Design review of the part built by this model. Coordinates are the model's own, in mm. A direction names the side the tool comes from. Coordinates: 2 decimals unless noted, no trailing zeros. Write each loop counter-clockwise with the first axis right and the second up, starting at its lowest first coordinate (ties: lowest second). Pieces come first, ordered by that corner, then holes. Notation, with made-up numbers: (44, 62.25) - (84, 62.25) arc R27 cw to (84, 81.25) - close; hole circle Ø6 at (17, 81). An arc over 180 degrees is marked (long way). Answer as a JSON object with one key per item and string values.
```python
from build123d import *

# Parameters (mm, degrees)
SKETCH_1_R          = 5.935
SKETCH_1_R_2        = 2.095
SKETCH_1_R_3        = 5.74
EXTRUDE_1_DEPTH     = 3.4
SKETCH_3_R          = 6.38
CUT_EXTRUDE_1_DEPTH = 2.9
SKETCH_4_R          = 4.5
EXTRUDE_3_DEPTH     = 0.56
SKETCH_6_R          = 3.15
CUT_EXTRUDE_2_DEPTH = 0.6
SKETCH_7_R          = 3.15
CUT_EXTRUDE_3_DEPTH = 0.6
SKETCH_8_R          = 3.15
CUT_EXTRUDE_4_DEPTH = 0.6
CUT_EXTRUDE_5_DEPTH = 10


with BuildPart() as part:
    # 草图1 → 凸台-拉伸1 (new body)
    # profile 1 of 4: a face of its own
    with BuildSketch(Plane.XY):
        with Locations((-32.939276233, 19.0175)):
            Circle(SKETCH_1_R)
        with Locations((-32.939276233, 19.0175)):
            Circle(SKETCH_1_R_2, mode=Mode.SUBTRACT)
    # profile 2 of 4: a face of its own
    with BuildSketch(Plane.XY):
        with Locations((32.939276233, 19.0175)):
            Circle(SKETCH_1_R)
        with Locations((32.939276233, 19.0175)):
            Circle(SKETCH_1_R_2, mode=Mode.SUBTRACT)
    # profile 3 of 4: a face of its own
    with BuildSketch(Plane.XY):
        with BuildLine():
            Line((-11.657112974, 15.201644655), (-30.328522818, 24.347433546))
            ThreePointArc((-30.328522818, 24.347433546), (-27.903452243, 22.158312274), (-27.004276233, 19.0175))
            ThreePointArc((-27.004276233, 19.0175), (-30.213751559, 13.745333439), (-36.370995778, 14.175235451))
            Line((-36.370995778, 14.175235451), (-17.779369394, 0.999324265))
            ThreePointArc((-17.779369394, 0.999324265), (-9.792356792, -8.015833705), (-6.620498611, -19.634988545))
            Line((-6.620498611, -19.634988545), (-5.935, -38.035))
            ThreePointArc((-5.935, -38.035), (0, -32.1), (5.935, -38.035))
            Line((5.935, -38.035), (6.620498611, -19.634988545))
            ThreePointArc((6.620498611, -19.634988545), (9.792356792, -8.015833705), (17.779369394, 0.999324265))
            Line((17.779369394, 0.999324265), (36.370995778, 14.175235451))
            ThreePointArc((36.370995778, 14.175235451), (27.836639672, 15.986439933), (30.328522818, 24.347433546))
            Line((30.328522818, 24.347433546), (11.657112974, 15.201644655))
            ThreePointArc((11.657112974, 15.201644655), (0, 12.5), (-11.657112974, 15.201644655))
        make_face()
        Circle(SKETCH_1_R_3, mode=Mode.SUBTRACT)
    # profile 4 of 4: a face of its own
    with BuildSketch(Plane.XY):
        with Locations((0, -38.035)):
            Circle(SKETCH_1_R)
        with Locations((0, -38.035)):
            Circle(SKETCH_1_R_2, mode=Mode.SUBTRACT)
    extrude(amount=EXTRUDE_1_DEPTH)

    # 草图3 → 切除-拉伸1 (cut)
    with BuildSketch(Plane(origin=(0, 0, 0), x_dir=(-1, 0, 0), z_dir=(0, 0, -1))):
        Circle(SKETCH_3_R)
    extrude(amount=-CUT_EXTRUDE_1_DEPTH, mode=Mode.SUBTRACT)

    # 草图4 → 凸台-拉伸3 (add)
    with BuildSketch(Plane(origin=(0, 0, 0), x_dir=(-1, 0, 0), z_dir=(0, 0, -1))):
        with Locations(Location((0, -38.035, 0), (0, 0, 180))):
            Circle(SKETCH_4_R)
        with Locations(Location((32.939276233, 19.0175, 0), (0, 0, 180))):
            Circle(SKETCH_4_R)
        with Locations(Location((-32.939276233, 19.0175, 0), (0, 0, 180))):
            Circle(SKETCH_4_R)
    extrude(amount=EXTRUDE_3_DEPTH)

    # 草图6 → 切除-拉伸2 (cut)
    with BuildSketch(Plane(origin=(0, 0, -0.56), x_dir=(-1, 0, 0), z_dir=(0, 0, -1))):
        with Locations((0, -38.035)):
            Circle(SKETCH_6_R)
    extrude(amount=-CUT_EXTRUDE_2_DEPTH, mode=Mode.SUBTRACT)

    # 草图7 → 切除-拉伸3 (cut)
    with BuildSketch(Plane(origin=(0, 0, -0.56), x_dir=(-1, 0, 0), z_dir=(0, 0, -1))):
        with Locations((-32.939276233, 19.0175)):
            Circle(SKETCH_7_R)
    extrude(amount=-CUT_EXTRUDE_3_DEPTH, mode=Mode.SUBTRACT)

    # 草图8 → 切除-拉伸4 (cut)
    with BuildSketch(Plane(origin=(0, 0, -0.56), x_dir=(-1, 0, 0), z_dir=(0, 0, -1))):
        with Locations((32.939276233, 19.0175)):
            Circle(SKETCH_8_R)
    extrude(amount=-CUT_EXTRUDE_4_DEPTH, mode=Mode.SUBTRACT)

    # 草图9 → 切除-旋转1 (revolve, cut)
    with BuildSketch(Plane(origin=(0, 19.0175, 0), x_dir=(-1, 0, 0), z_dir=(0, -1, 0))):
        Polygon((35.034276233, -3.4), (35.034276233, -1.425), (37.009276233, -3.4), align=None)
    revolve(axis=Axis((-32.939276233, 19.0175, 3.4), (0, 0, -1)), mode=Mode.SUBTRACT)

    # 草图10 → 切除-旋转2 (revolve, cut)
    with BuildSketch(Plane(origin=(16.469638116, -9.50875, 0), x_dir=(0, 0, 1), z_dir=(-0.8660254037844397, 0.49999999999999806, 0)), mode=Mode.PRIVATE) as cut_revolve_2_sk:
        Polygon((3.4, 35.034276233), (3.4, 37.009276233), (1.425, 35.034276233), align=None)
    revolve(cut_revolve_2_sk.sketch.rotate(Axis((32.939276233, 19.0175, 3.4), (0, 0, -1)), 240), axis=Axis((32.939276233, 19.0175, 3.4), (0, 0, -1)), mode=Mode.SUBTRACT)

    # 草图11 → 切除-旋转3 (revolve, cut)
    with BuildSketch(Plane(origin=(16.469638116, -9.50875, 0), x_dir=(0, 0, 1), z_dir=(-0.8660254037844397, 0.49999999999999806, 0)), mode=Mode.PRIVATE) as cut_revolve_3_sk:
        Polygon((3.4, -30.844276233), (3.4, -28.869276233), (1.425, -30.844276233), align=None)
    revolve(cut_revolve_3_sk.sketch.rotate(Axis((0, -38.035, 3.4), (0, 0, -1)), 240), axis=Axis((0, -38.035, 3.4), (0, 0, -1)), mode=Mode.SUBTRACT)

    # 草图12 → 切除-拉伸5 (cut)
    with BuildSketch(Plane(origin=(0, 0, 0), x_dir=(-1, 0, 0), z_dir=(0, 0, -1))):
        with BuildLine():
            Line((-4.991404318, -9.920918283), (-4.002436423, -30.667860961))
            ThreePointArc((-4.002436423, -30.667860961), (-3.542480946, -31.462610037), (-2.628124289, -31.547091036))
            ThreePointArc((-2.628124289, -31.547091036), (-0.124699507, -31.0361108), (2.395338905, -31.457587778))
            ThreePointArc((2.395338905, -31.457587778), (3.286322012, -31.353916504), (3.73574796, -30.577633728))
            Line((3.73574796, -30.577633728), (4.96942943, -9.941577808))
            ThreePointArc((4.96942943, -9.941577808), (4.555657168, -9.070468591), (3.598327924, -8.954023462))
            ThreePointArc((3.598327924, -8.954023462), (-0.010417716, -9.649994377), (-3.617652266, -8.946233402))
            ThreePointArc((-3.617652266, -8.946233402), (-4.57119236, -9.057730973), (-4.991404318, -9.920918283))
        make_face()
        with BuildLine():
            Line((-6.096065103, 9.283142082), (-24.55792846, 18.8001421))
            ThreePointArc((-24.55792846, 18.8001421), (-25.476179088, 18.79918351), (-26.006520108, 18.049567917))
            ThreePointArc((-26.006520108, 18.049567917), (-26.815710634, 15.626048341), (-28.44073961, 13.654369547))
            ThreePointArc((-28.44073961, 13.654369547), (-28.796449207, 12.830919904), (-28.348881576, 12.053564228))
            Line((-28.348881576, 12.053564228), (-11.09437365, 0.667136775))
            ThreePointArc((-11.09437365, 0.667136775), (-10.133084808, 0.589919457), (-9.553575746, 1.360768338))
            ThreePointArc((-9.553575746, 1.360768338), (-8.351931419, 4.834019195), (-5.938839262, 7.606095465))
            ThreePointArc((-5.938839262, 7.606095465), (-5.558628943, 8.487634196), (-6.096065103, 9.283142082))
        make_face()
        with BuildLine():
            Line((11.087469421, 0.637776201), (28.560364883, 11.867718861))
            ThreePointArc((28.560364883, 11.867718861), (29.018660034, 12.663426527), (28.634644397, 13.49752312))
            ThreePointArc((28.634644397, 13.49752312), (26.940410141, 15.410062459), (26.045400706, 17.803218231))
            ThreePointArc((26.045400706, 17.803218231), (25.510127195, 18.5229966), (24.613133616, 18.5240695))
            Line((24.613133616, 18.5240695), (6.12494422, 9.274441032))
            ThreePointArc((6.12494422, 9.274441032), (5.57742764, 8.480549134), (5.955247822, 7.593255124))
            ThreePointArc((5.955247822, 7.593255124), (8.362349135, 4.815975182), (9.556491527, 1.340137937))
            ThreePointArc((9.556491527, 1.340137937), (10.129821304, 0.570096777), (11.087469421, 0.637776201))
        make_face()
    extrude(amount=-CUT_EXTRUDE_5_DEPTH, mode=Mode.SUBTRACT)


solid = part.part
```
(1) To check wall thickness, follow line 1 (X direction, y = 8, z = 2.6); line 2 (X direction, y = 10.5, z = 0.45); line 3 (Y direction, x = 3, z = 2.6). State the ranges of each line that lie inside material, in increasing order. Write a range as from..to.
Solved:
{"line 1": "x = -27.66..-22.54, -5.65..5.64, 22.21..27.66", "line 2": "x = -31.19..-26.43, -8.57..8.46, 25.99..31.19", "line 3": "y = -43.16..-39.34, -36.73..-31.62, -9.17..-5.63, 5.63..12.67"}
(2) Take a section at D-D, the plane y = -17.5. Write out the cut boundary in (x, z), and give its area (3 significant figures).
Solved:
{"outline": "(-6.79, 0) - (-4.52, 0) - (-4.52, 3.4) - (-6.79, 3.4) - close; (4.63, 0) - (6.79, 0) - (6.79, 3.4) - (4.63, 3.4) - close", "area": "15.0 mm^2"}
(3) Tool access review of faces 1 (the face through (6, 1, 2.9)), 2 (the face through (-31.304, 20.517, 1.549)), 3 (the face through (-20.86, 19.71, 1.68)), 4 (the face through (-5.58, 8.49, 1.68)): name each direction out of +Z, -Z, +X, -X, +Y, -Y from which nothing blocks a thin tool from reaching the whole face with its end or side.
Solved:
{"face 1": "-Z", "face 2": "+Z", "face 3": "+Z, -Z, +Y", "face 4": "+Z, -Z"}
(4) Take a section at C-C, the plane x = -12.5. Write out the cut boundary in (y, z), and give its area (3 significant figures).
Solved:
{"outline": "(-3.95, 0) - (1.55, 0) - (1.55, 3.4) - (-3.95, 3.4) - close; (12.46, 0) - (15.61, 0) - (15.61, 3.4) - (12.46, 3.4) - close", "area": "29.4 mm^2"}
(5) The part is to be moulded in two halves that separate along X. For faces 5 (the face through (9.71, -8.17, 1.68)), 6 (the face through (-8.336, 4.861, 1.676)), 7 (the face through (-6, 1, 3.4)), 8 (the face through (-36.51, 21.756, -0.276)), say which applies: pulls with the +X half, pulls with the -X half, needs draft (parallel to the pull), parting line crosses it, or undercut.
Solved:
{"face 5": "pulls with the +X half", "face 6": "undercut", "face 7": "needs draft", "face 8": "undercut"}
(6) Take a section at A-A, the plane x = 0. Give the number of separate pieces and of enclosed holes in the cut face, and give its area (3 significant figures).
Solved:
{"separate pieces": "4", "enclosed holes": "0", "area": "59.8 mm^2"}
(7) Take a section at B-B, the plane y = 3.5. Write out the cut boundary in (x, z), and give its area (3 significant figures).
Solved:
{"outline": "(-21.31, 0) - (-15.54, 0) - (-15.54, 3.4) - (-21.31, 3.4) - close; (-8.99, 0) - (-5.33, 0) - (-5.33, 2.9) - (-4.55, 2.9) - (-4.55, 3.4) - (-8.99, 3.4) - close; (4.55, 2.9) - (5.33, 2.9) - (5.33, 0) - (8.99, 0) - (8.99, 3.4) - (4.55, 3.4) - close; (15.39, 0) - (21.31, 0) - (21.31, 3.4) - (15.39, 3.4) - close", "area": "65.4 mm^2"}
(8) For pin 1 (10.5 mm diameter, centred on x = 0, y = 0, fed in from +Z); pin 2 (14 mm diameter, centred on x = 0, y = -2.5, fed in from -Z); pin 3 (1 mm diameter, centred on y = -35.5, z = 3, fed in from -X), all flat-tipped, find the tip position at first contact; note any pin that passes through.
Solved:
{"pin 1": "passes through", "pin 2": "stops at z = 0", "pin 3": "stops at x = -6.05"}
